Geometry check sheet. Reference: the model listing, model coordinates, mm. A direction names the side the tool comes from. Round coordinates to 2 decimals unless told otherwise and drop trailing zeros. Write each loop counter-clockwise with the first axis right and the second up, starting at its lowest first coordinate (ties: lowest second). Pieces come first, ordered by that corner, then holes. Notation, with made-up numbers: M 39,76 L 83,76 A6 cw 83,87 Z; hole C 61,38.25 d5. An arc over 180 degrees is marked long. Put each result on its own line as item: value. Start each with the question number.
(1) Section check B-B on z = 5. Record the cut outline in (x, y).
(2) Section check A-A on x = -80.5. Record the cut outline in (y, z), then the cut area to 3 significant figures.
(3) Tool access check on faces 1 (the flat face through (-38.32, -0.069, 2.028)), 2 (the flat face through (-99.549, 0, 11)), 3 (the flat face through (-50, 0, 22)), 4 (the flat face through (-89, 3, 0)), 5 (the flat face through (-54, 4.897, 11)). Record the directions out of +Z, -Z, +X, -X, +Y, -Y that give a thin tool (end or side, any length) a straight path to the whole face; none if there is none.
(4) Material ranges on probe 1 along X at (y, z) = (0.25, 8); probe 2 along Y at (x, z) = (-82, 17.25); probe 3 along Y at (x, z) = (0, 14), recorded low to high.
(5) Mould release check, pull along Y, two halves, no side actions. Record for faces 6 (the flat face through (-75.338, 0, 11)), 7 (the flat face through (-55, -4.897, 11)), 8 (the cylindrical face through (-107.483, 0.124, 10.846)): pulls with the +Y half, pulls with the -Y half, needs draft (parallel to the pull), parting line crosses it, or undercut.
(6) Section check C-C on y = 0. Record the cut outline in (x, z).
(7) Section check D-D on x = 0. Record the cut outline in (y, z), then the cut area to 3 significant figures.
(8) Gauge pin test, flat ends, axial feed: pin 1 (3 mm diameter, centred on y = 3, z = 12, fed in from -X); pin 2 (8 mm diameter, centred on y = -6, z = 5.5, fed in from -X); pin 3 (8 mm diameter, centred on x = -56, z = 20, fed in from +Y); pin 4 (8 mm diameter, centred on x = -42, y = 7, fed in from +Z). Record the tip position at first contact, or that the pin passes through.
from build123d import *

# Parameters (mm, degrees)
F1_DEPTH = 22
F3_DEPTH = 13.5984562425
F4_W     = 24.2116302252
F4_H     = 2.5544243399
F4_H_2   = 2.1986933425
F5_DEPTH = 22.001
F6_R     = 4.0024769444
F7_DEPTH = 22.001


with BuildPart() as f1:
    # F0 (on Top) → F1 (new body)
    with BuildSketch(Plane.XY):
        with BuildLine():
            Line((-101.4767971394, -4.8974562425), (-7.1906134893, -4.8974562425))
            ThreePointArc((-7.1906134893, -4.8974562425), (8.7, 0), (-7.1906134893, 4.8974562425))
            Line((-7.1906134893, 4.8974562425), (-101.4767971394, 4.8974562425))
            ThreePointArc((-101.4767971394, 4.8974562425), (-107.4842306869, 0), (-101.4767971394, -4.8974562425))
        make_face()
    extrude(amount=F1_DEPTH)

    # F2 (on face) → F3 (cut, through all)
    with BuildSketch(Plane.XZ.offset(4.8974562425)):
        Polygon((-7.1906134893, 3.9995550178), (-70.3336670995, 0), (-7.1906134893, 0), align=None)
    extrude(amount=-F3_DEPTH, mode=Mode.SUBTRACT)

    # F4 (on face) → F5 (cut, through all)
    with BuildSketch(Plane.XY.offset(22)):
        with Locations((-87.4435827136, 1.27721217)):
            Rectangle(F4_W, F4_H)
        with Locations((-87.4435827136, -1.0993466713)):
            Rectangle(F4_W, F4_H_2)
    extrude(amount=-F5_DEPTH, mode=Mode.SUBTRACT)

    # F6 (on face) → F7 (cut, through all)
    with BuildSketch(Plane.XY.offset(22)):
        Circle(F6_R)
    extrude(amount=-F7_DEPTH, mode=Mode.SUBTRACT)


solid = f1.part
Answers follow:
1. outline: M -101.48,-4.9 L -7.19,-4.9 A8.7 ccw long -7.19,4.9 L -101.48,4.9 A5 ccw long Z; hole M -99.55,-2.2 L -75.34,-2.2 L -75.34,2.55 L -99.55,2.55 Z; hole C 0,0 d8
2. outline: M -4.9,0 L -2.2,0 L -2.2,22 L -4.9,22 Z; M 2.55,0 L 4.9,0 L 4.9,22 L 2.55,22 Z
2. area: 111 mm^2
3. face 1: -Z, +Y, -Y
3. face 2: +Z, -Z
3. face 3: +Z, +X, -X, +Y, -Y
3. face 4: -Z, +X, -X, +Y, -Y
3. face 5: +Z, -Z, +Y
4. probe 1: x = -107.48 to -99.55, -75.34 to -3.99, 3.99 to 8.7
4. probe 2: y = -4.9 to -2.2, 2.55 to 4.9
4. probe 3: y = -8.7 to -4, 4 to 8.7
5. face 6: undercut
5. face 7: pulls with the -Y half
5. face 8: parting line crosses it
6. outline: M -107.48,0 L -99.55,0 L -99.55,22 L -107.48,22 Z; M -75.34,0 L -70.33,0 L -7.19,4 L -7.19,0 L -4,0 L -4,22 L -75.34,22 Z; M 4,0 L 8.7,0 L 8.7,22 L 4,22 Z
7. outline: M -8.7,0 L -4,0 L -4,22 L -8.7,22 Z; M 4,0 L 8.7,0 L 8.7,22 L 4,22 Z
7. area: 207 mm^2
8. pin 1: stops at x = -107.25
8. pin 2: stops at x = -107.07
8. pin 3: stops at y = 4.9
8. pin 4: stops at z = 22
